Input: part model. Units: mm. Frame: model coordinates. Face numbers are marked on the shaded views. A direction names the side the tool comes from. Coordinates: 2 decimals unless noted, no trailing zeros. Write each loop counter-clockwise with the first axis right and the second up, starting at its lowest first coordinate (ties: lowest second). Pieces come first, ordered by that corner, then holes. Notation, with made-up numbers: (23, 4) - (70, 4) arc R21 cw to (70, 31) - close; hole circle Ø7 at (85.25, 84). An arc over 180 degrees is marked (long way). Use a Markdown table: item, result. Add a question column.
Q1. Section query C-C (z = -5). Return the cut outline in (x, y).
Q2. Mould query, pull axis X, two halves, no side actions, for the marked faces 1, 2 and 3. Classes: released by +X, released by -X, zero draft, split by the parting line, or undercut.
Q3. Set-up query: the marked faces 4 and 5. Return all of +Z, -Z, +X, -X, +Y, -Y with unobstructed straight access to the full face (end or side cutting, diameter ignored); none if empty.
Q4. Pin query (flat end, axial travel): P1, Ø8, axis at x = -2.5, y = 30, coming from the -Z side; P2, Ø2, axis at x = -5, z = 6.5, coming from the +Y side; P3, Ø0.9, axis at x = 11, y = 40.5, coming from the -Z side; P4, Ø0.5, axis at x = 8.5, y = 39, coming from the +Z side. Return the tip coordinate at first contact, or that it passes through.
Q5. Section query B-B (y = 28). Return the cut outline in (x, z), then the cut area to 3 significant figures.
Q6. Section query D-D (z = -1.75). Return the cut outline in (x, y).
Q7. Material intervals for probe 1 along X at (y, z) = (33, 11.25); probe 2 along Y at (x, z) = (-6.5, 10); probe 3 along Y at (x, z) = (-9.5, 8.5), sorted ascending. Write a range as from..to.
from build123d import *

# Parameters (mm, degrees)
SKETCH1_W           = 25.4
SKETCH1_H           = 25.4
BOSS_EXTRUDE1_DEPTH = 50.8
SKETCH2_W           = 13.208
SKETCH2_H           = 25.4
CUT_EXTRUDE1_DEPTH  = 38.1
CUT_EXTRUDE2_DEPTH  = 59.198711326
FILLET1_R           = 12.7


with BuildPart() as part:
    # Sketch1 → Boss-Extrude1 (new body)
    with BuildSketch(Plane(origin=(0, 0, 0), x_dir=(1, 0, 0), z_dir=(0, 1, 0))):
        Rectangle(SKETCH1_W, SKETCH1_H)
    extrude(amount=BOSS_EXTRUDE1_DEPTH)

    # Sketch2 → Cut-Extrude1 (cut)
    with BuildSketch(Plane(origin=(0, 50.8, 0), x_dir=(1, 0, 0), z_dir=(0, 1, 0))):
        Rectangle(SKETCH2_W, SKETCH2_H)
    extrude(amount=-CUT_EXTRUDE1_DEPTH, mode=Mode.SUBTRACT)

    # Sketch3 → Cut-Extrude2 (cut, through all)
    with BuildSketch(Plane(origin=(12.7, 0, 0), x_dir=(0, 0, -1), z_dir=(1, 0, 0))):
        Polygon((-0.889, 41.312023576), (0.889, 41.312023576), (0.889, 39.534023576), (2.667, 39.534023576), (2.667, 37.756023576), (0.889, 37.756023576), (0.889, 35.978023576), (-0.889, 35.978023576), (-0.889, 37.756023576), (-2.667, 37.756023576), (-2.667, 39.534023576), (-0.889, 39.534023576), align=None)
    extrude(amount=-CUT_EXTRUDE2_DEPTH, mode=Mode.SUBTRACT)

    # Fillet1
    fillet1_edges = [part.edges().sort_by_distance(p)[0] for p in [
        (9.652, 50.8, -12.7),
        (-9.652, 50.8, -12.7),
        (-9.652, 50.8, 12.7),
        (9.652, 50.8, 12.7),
    ]]
    fillet(fillet1_edges, radius=FILLET1_R - 0.0001)  # a hair under: the kernel refuses the full size


solid = part.part
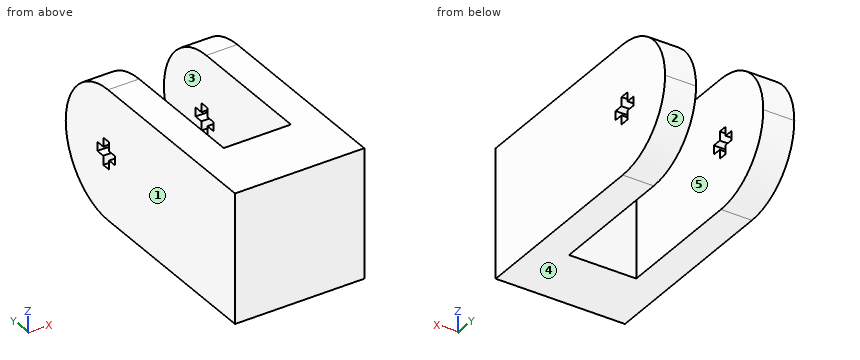
Values follow:
| question | item | result |
|---|---|---|
| 1 | outline | (-12.7, 0) - (12.7, 0) - (12.7, 49.77) - (6.6, 49.77) - (6.6, 12.7) - (-6.6, 12.7) - (-6.6, 49.77) - (-12.7, 49.77) - close |
| 2 | face 1 | released by -X |
| 2 | face 2 | zero draft |
| 2 | face 3 | undercut |
| 3 | face 4 | -Z, +X, -X, +Y, -Y |
| 3 | face 5 | +Z, -Z, +Y |
| 4 | P1 | through |
| 4 | P2 | y = 12.7 |
| 4 | P3 | z = -12.55 |
| 4 | P4 | z = 12.68 |
| 5 | outline | (-12.7, -12.7) - (-6.6, -12.7) - (-6.6, 12.7) - (-12.7, 12.7) - close; (6.6, -12.7) - (12.7, -12.7) - (12.7, 12.7) - (6.6, 12.7) - close |
| 5 | area | 310 mm2 |
| 6 | outline | (-12.7, 0) - (12.7, 0) - (12.7, 37.76) - (6.6, 37.76) - (6.6, 12.7) - (-6.6, 12.7) - (-6.6, 37.76) - (-12.7, 37.76) - close; (-12.7, 39.53) - (-6.6, 39.53) - (-6.6, 50.68) - (-12.7, 50.68) - close; (6.6, 39.53) - (12.7, 39.53) - (12.7, 50.68) - (6.6, 50.68) - close |
| 7 | probe 1 | -12.7..-6.6, 6.6..12.7 |
| 7 | probe 2 | 0..12.7 |
| 7 | probe 3 | 0..47.54 |
